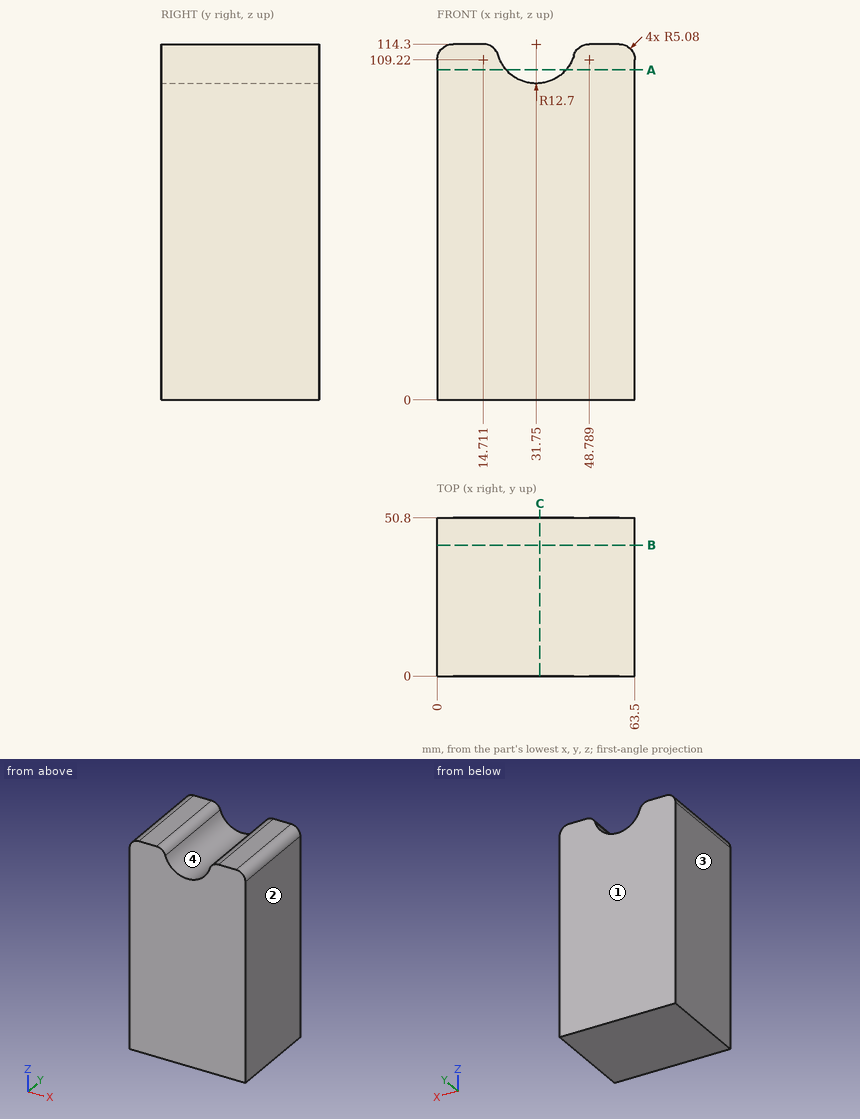
Job drawing, mm, ordinate dimensions from the low corner. One solid piece. Round coordinates to 2 decimals unless told otherwise and drop trailing zeros. Order: outer loops, then holes, each group sorted by start corner. A loop starts at its lowest first (then second) coordinate and runs counter-clockwise, first axis right, second up. Notation, with made-up numbers: (-27.75, 53) -> (-16.75, 53) arc R27 ccw to (-16.75, 73) -> close; hole circle Ø9 at (73, 29.5). An arc over 180 degrees is marked (long way). Write item = value, one per line.
(1) Cut at C-C (x = 33). Write the cut outline in (y, z), plus the area to 3 significant figures.
Answers follow:
outline = (0, 0) -> (50.8, 0) -> (50.8, 101.66) -> (0, 101.66) -> close
area = 5,160 mm²
(2) Drill centre lines: L1, parallel to X at y = 47, z = 106.5; L2, parallel to Z at x = 29, y = 48; L3, parallel to Z at x = 38.5, y = 5. Where is each one in solid material? Low to high.
Answers follow:
L1 = 0 to 21.73, 41.77 to 63.5
L2 = 0 to 101.9
L3 = 0 to 103.54
(3) Pull direction X, two halves, no side cores. Call the marked faces 1, 2, 3 and 4: +X half, -X half, draft (parallel to the pull), parting line (faces both ways), or undercut.
Answers follow:
face_1 = draft
face_2 = +X half
face_3 = -X half
face_4 = undercut
(4) Flat gauge pins, fed straight in: P1, Ø2, axis at x = 41, y = 37.5, coming from the +Z side; P2, Ø2, axis at x = 17, y = 40.5, coming from the +Z side. Where does each tip first touch, or does it go through?
Answers follow:
P1 = 106.8
P2 = 114.13
(5) Cut at B-B (y = 42). Write the cut outline in (x, z), plus the area to 3 significant figures.
Answers follow:
outline = (0, 0) -> (63.5, 0) -> (63.5, 109.22) arc R5.08 ccw to (58.42, 114.3) -> (48.79, 114.3) arc R5.08 ccw to (43.92, 110.67) arc R12.7 cw to (19.58, 110.67) arc R5.08 ccw to (14.71, 114.3) -> (5.08, 114.3) arc R5.08 ccw to (0, 109.22) -> close
area = 6,990 mm²
(6) Cut at A-A (z = 106). Write the cut outline in (x, y).
Answers follow:
outline = (0, 0) -> (22.14, 0) -> (22.14, 50.8) -> (0, 50.8) -> close; (41.36, 0) -> (63.5, 0) -> (63.5, 50.8) -> (41.36, 50.8) -> close
